from build123d import *

# Parameters (mm, degrees)
SKETCH1_W           = 42
SKETCH1_H           = 15
BOSS_EXTRUDE1_DEPTH = 5
SKETCH2_R           = 1.115
CUT_EXTRUDE1_DEPTH  = 6
SKETCH3_W           = 15
SKETCH3_H           = 80.5
BOSS_EXTRUDE2_DEPTH = 5
SKETCH4_W           = 35
SKETCH4_H           = 10
BOSS_EXTRUDE3_DEPTH = 5
SKETCH5_W           = 10
SKETCH5_H           = 10
BOSS_EXTRUDE4_DEPTH = 5
SKETCH6_R           = 1.75
CUT_EXTRUDE2_DEPTH  = 6
SKETCH7_W           = 15
SKETCH7_H           = 0.2
CUT_EXTRUDE3_DEPTH  = 6
SKETCH8_W           = 2
SKETCH8_H           = 105.3
BOSS_EXTRUDE5_DEPTH = 10
CUT_EXTRUDE4_DEPTH  = 23


with BuildPart() as part:
    # Sketch1 → Boss-Extrude1 (new body)
    with BuildSketch(Plane(origin=(0, 0, 0), x_dir=(1, 0, 0), z_dir=(0, 1, 0))):
        with Locations((21, 7.5)):
            Rectangle(SKETCH1_W, SKETCH1_H)
    extrude(amount=BOSS_EXTRUDE1_DEPTH)

    # Sketch2 → Cut-Extrude1 (cut, through all)
    with BuildSketch(Plane(origin=(0, 5, 0), x_dir=(1, 0, 0), z_dir=(0, 1, 0))):
        with Locations((3, 7.5)):
            Circle(SKETCH2_R)
        with Locations((39, 7.5)):
            Circle(SKETCH2_R)
    extrude(amount=-CUT_EXTRUDE1_DEPTH, mode=Mode.SUBTRACT)

    # Sketch3 → Boss-Extrude2 (add)
    with BuildSketch(Plane(origin=(0, 5, 0), x_dir=(1, 0, 0), z_dir=(0, 1, 0))):
        with Locations((21, -40.25)):
            Rectangle(SKETCH3_W, SKETCH3_H)
    extrude(amount=-BOSS_EXTRUDE2_DEPTH)

    # Sketch4 → Boss-Extrude3 (add)
    with BuildSketch(Plane(origin=(0, 5, 0), x_dir=(1, 0, 0), z_dir=(0, 1, 0))):
        with Locations((21, -85.5)):
            Rectangle(SKETCH4_W, SKETCH4_H)
    extrude(amount=-BOSS_EXTRUDE3_DEPTH)

    # Sketch5 → Boss-Extrude4 (add)
    with BuildSketch(Plane(origin=(0, 5, 0), x_dir=(1, 0, 0), z_dir=(0, 1, 0))):
        with Locations((8.5, -95.5)):
            Rectangle(SKETCH5_W, SKETCH5_H)
        with Locations((33.5, -95.5)):
            Rectangle(SKETCH5_W, SKETCH5_H)
    extrude(amount=-BOSS_EXTRUDE4_DEPTH)

    # Sketch6 → Cut-Extrude2 (cut, through all)
    with BuildSketch(Plane(origin=(0, 5, 0), x_dir=(1, 0, 0), z_dir=(0, 1, 0))):
        with Locations((8.5, -95.5)):
            Circle(SKETCH6_R)
        with Locations((33.5, -95.5)):
            Circle(SKETCH6_R)
    extrude(amount=-CUT_EXTRUDE2_DEPTH, mode=Mode.SUBTRACT)

    # Sketch7 → Cut-Extrude3 (cut, through all)
    with BuildSketch(Plane(origin=(0, 5, 0), x_dir=(1, 0, 0), z_dir=(0, 1, 0))):
        with Locations((21, -90.4)):
            Rectangle(SKETCH7_W, SKETCH7_H)
    extrude(amount=-CUT_EXTRUDE3_DEPTH, mode=Mode.SUBTRACT)

    # Sketch8 → Boss-Extrude5 (add)
    with BuildSketch(Plane(origin=(0, 5, 0), x_dir=(1, 0, 0), z_dir=(0, 1, 0))):
        with Locations((21, -37.65)):
            Rectangle(SKETCH8_W, SKETCH8_H)
    extrude(amount=BOSS_EXTRUDE5_DEPTH)

    # Sketch9 → Cut-Extrude4 (cut, through all)
    with BuildSketch(Plane.ZY.offset(-20)):
        Polygon((-15, 15), (90.5, 5), (90.3, 15), align=None)
    extrude(amount=-CUT_EXTRUDE4_DEPTH, mode=Mode.SUBTRACT)


solid = part.part
Here's how the part is built. I have some questions about the finished solid (model axes, mm). A direction names the side the tool comes from. Round coordinates to 2 decimals unless told otherwise and drop trailing zeros. Write each loop counter-clockwise with the first axis right and the second up, starting at its lowest first coordinate (ties: lowest second). Pieces come first, ordered by that corner, then holes.
1. Suppose I cut it at D-D (x = 8.5). List the corners of the cut face in (y, z) for me, and give its area (4 significant figures).
2. For faces 1 (the flat face through (7, 2, 0)), 2 (the flat face through (33, 3, 80.5)), 3 (the flat face through (14, 5, 29)), which set-ups out of +Z, -Z, +X, -X, +Y, -Y let a thin tool reach every point of the face, with its end or its side?
3. Suppose I cut it at B-B (z = 95.5). List the corners of the cut face in (x, y) for me, and give its area (3 significant figures).
4. Will these pins go through, and if not, where does the flat tip stop? pin 1 Ø4.5 at (x, z) = (33.5, 95.5) entering from +Y; pin 2 Ø1.5 at (y, z) = (1.5, 58) entering from +X; pin 3 Ø2.5 at (y, z) = (2.5, 91.5) entering from +X; pin 4 Ø1.3 at (x, z) = (3, -7.5) entering from +Y.
5. Suppose I cut it at A-A (x = 29.5). List the corners of the cut face in (y, z) for me.
6. Suppose I cut it at C-C (y = 2). List the corners of the cut face in (x, z) for me (3 decimals), and give its area (3 significant figures).
7. If we mould it in two halves opening along X, with no side actions, what happens to faces 4 (the flat face through (21, 0, 29)), 5 (the flat face through (21, 3, 90.3)), 6 (the flat face through (3.5, 3, 91))? For each: released by +X, released by -X, zero draft, split by the parting line, or undercut.
8. I need wall thicknesses on L1, parallel to X at y = 2.55, z = 95.5; L2, parallel to Z at x = 8.5, y = 1.8; L3, parallel to X at y = 1.15, z = -7.5 (3 decimals). Which ranges of each line are inside material? Lowest first, please.
Answer sheet:
1. outline: (0, -15) - (5, -15) - (5, 0) - (0, 0) - close; (0, 80.5) - (5, 80.5) - (5, 93.75) - (0, 93.75) - close; (0, 97.25) - (5, 97.25) - (5, 100.5) - (0, 100.5) - close
1. area: 157.5 mm2
2. face 1: -X, +Y, -Y
2. face 2: +X, +Y, -Y
2. face 3: +Z, -Z, -X, +Y
3. outline: (3.5, 0) - (6.75, 0) - (6.75, 5) - (3.5, 5) - close; (10.25, 0) - (13.5, 0) - (13.5, 5) - (10.25, 5) - close; (28.5, 0) - (31.75, 0) - (31.75, 5) - (28.5, 5) - close; (35.25, 0) - (38.5, 0) - (38.5, 5) - (35.25, 5) - close
3. area: 65.0 mm2
4. pin 1: stops at y = 5
4. pin 2: stops at x = 28.5
4. pin 3: stops at x = 38.5
4. pin 4: passes through
5. outline: (0, -15) - (5, -15) - (5, 0) - (0, 0) - close; (0, 80.5) - (5, 80.5) - (5, 100.5) - (0, 100.5) - close
6. outline: (0, -15) - (42, -15) - (42, 0) - (28.5, 0) - (28.5, 80.5) - (38.5, 80.5) - (38.5, 100.5) - (28.5, 100.5) - (28.5, 90.3) - (13.5, 90.3) - (13.5, 100.5) - (3.5, 100.5) - (3.5, 80.5) - (13.5, 80.5) - (13.5, 0) - (0, 0) - close; hole circle Ø2.23 at (3, -7.5); hole circle Ø3.5 at (8.5, 95.5); hole circle Ø3.5 at (33.5, 95.5); hole circle Ø2.23 at (39, -7.5)
6. area: 2,360 mm2
7. face 4: zero draft
7. face 5: undercut
7. face 6: released by -X
8. L1: x = 3.5 to 6.75, 10.25 to 13.5, 28.5 to 31.75, 35.25 to 38.5
8. L2: z = -15 to 0, 80.5 to 93.75, 97.25 to 100.5
8. L3: x = 0 to 1.885, 4.115 to 37.885, 40.115 to 42
